```python
from build123d import *

# Parameters (mm, degrees)
BOSS_EXTRUDE1_DEPTH      = 115
CUT_EXTRUDE3_START       = -15
CUT_EXTRUDE3_DEPTH       = 15
CUT_EXTRUDE4_DEPTH       = 67
SKETCH5_W                = 33
SKETCH5_H                = 40
CUT_EXTRUDE5_DEPTH       = 67
SKETCH6_W                = 40
SKETCH6_H                = 15
BOSS_EXTRUDE2_DEPTH      = 5
SKETCH7_W                = 15
SKETCH7_H                = 15
BOSS_EXTRUDE4_DEPTH      = 10
SKETCH8_W                = 7
SKETCH8_H                = 15
BOSS_EXTRUDE5_DEPTH      = 5
BOSS_EXTRUDE6_DEPTH      = 5
BOSS_EXTRUDE6_DEPTH_BACK = 15
SKETCH9_W                = 40
SKETCH9_H                = 15


with BuildPart() as part:
    # Sketch1 → Boss-Extrude1 (new body)
    with BuildSketch(Plane(origin=(0, 0, 0), x_dir=(0, 0, -1), z_dir=(1, 0, 0))):
        with BuildLine():
            Line((-10, 54.083269132), (-10, -1.916730868))
            ThreePointArc((-10, -1.916730868), (-7.071067812, -8.98779868), (0, -11.916730868))
            Line((0, -11.916730868), (20, -11.916730868))
            Line((20, -11.916730868), (20, -26.916730868))
            Line((20, -26.916730868), (-20, -26.916730868))
            Line((-20, -26.916730868), (-20, -51.23475383))
            ThreePointArc((-20, -51.23475383), (-54.753734942, 5.198895061), (-10, 54.083269132))
        make_face()
    extrude(amount=BOSS_EXTRUDE1_DEPTH)

    # Sketch2 → Cut-Extrude3 (cut)
    with BuildSketch(Plane(origin=(115, 0, 0), x_dir=(0, 0, -1), z_dir=(1, 0, 0)).offset(CUT_EXTRUDE3_START)):
        with BuildLine():
            Line((20, -21.916730868), (-54.666698166, -6.045834235))
            ThreePointArc((-54.666698166, -6.045834235), (-45.878767393, 34.080884973), (-10, 54.083269132))
            Line((-10, 54.083269132), (-10, -1.916730868))
            ThreePointArc((-10, -1.916730868), (-7.071067812, -8.98779868), (0, -11.916730868))
            Line((0, -11.916730868), (20, -11.916730868))
            Line((20, -11.916730868), (20, -21.916730868))
        make_face()
    extrude(amount=CUT_EXTRUDE3_DEPTH, mode=Mode.SUBTRACT)

    # Sketch4 → Cut-Extrude4 (cut)
    with BuildSketch(Plane(origin=(0, -11.916730868, 0), x_dir=(1, 0, 0), z_dir=(0, 1, 0))):
        with BuildLine():
            Line((10, 15), (90, 15))
            ThreePointArc((90, 15), (95, 10), (90, 5))
            Line((90, 5), (10, 5))
            ThreePointArc((10, 5), (5, 10), (10, 15))
        make_face()
    extrude(amount=-CUT_EXTRUDE4_DEPTH, mode=Mode.SUBTRACT)

    # Sketch5 → Cut-Extrude5 (cut)
    with BuildSketch(Plane(origin=(0, 0, 10), x_dir=(-1, 0, 0), z_dir=(0, 0, -1))):
        with Locations((-53.5, 34.083269132)):
            Rectangle(SKETCH5_W, SKETCH5_H)
    extrude(amount=-CUT_EXTRUDE5_DEPTH, mode=Mode.SUBTRACT)

    # Sketch6 → Boss-Extrude2 (add)
    with BuildSketch(Plane(origin=(0, 0, 10), x_dir=(-1, 0, 0), z_dir=(0, 0, -1))):
        with Locations((-17, 31.583269132)):
            Rectangle(SKETCH6_W, SKETCH6_H)
    extrude(amount=BOSS_EXTRUDE2_DEPTH)

    # Sketch7 → Boss-Extrude4 (add)
    with BuildSketch(Plane.ZY):
        with Locations((17.5, 31.583269132)):
            Rectangle(SKETCH7_W, SKETCH7_H)
    extrude(amount=BOSS_EXTRUDE4_DEPTH)

    # Sketch8 → Boss-Extrude5 (add)
    with BuildSketch(Plane(origin=(0, 0, 10), x_dir=(-1, 0, 0), z_dir=(0, 0, -1))):
        with Locations((6.5, 31.583269132)):
            Rectangle(SKETCH8_W, SKETCH8_H)
    extrude(amount=BOSS_EXTRUDE5_DEPTH)

    # Sketch9 → Boss-Extrude6 (add, two sides: drawn at the far end of the back side and taken through both)
    with BuildSketch(Plane(origin=(0, 0, 10), x_dir=(-1, 0, 0), z_dir=(0, 0, -1)).offset(-BOSS_EXTRUDE6_DEPTH_BACK)):
        with Locations((-90, 31.583269132)):
            Rectangle(SKETCH9_W, SKETCH9_H)
    extrude(amount=BOSS_EXTRUDE6_DEPTH + BOSS_EXTRUDE6_DEPTH_BACK)


solid = part.part
```
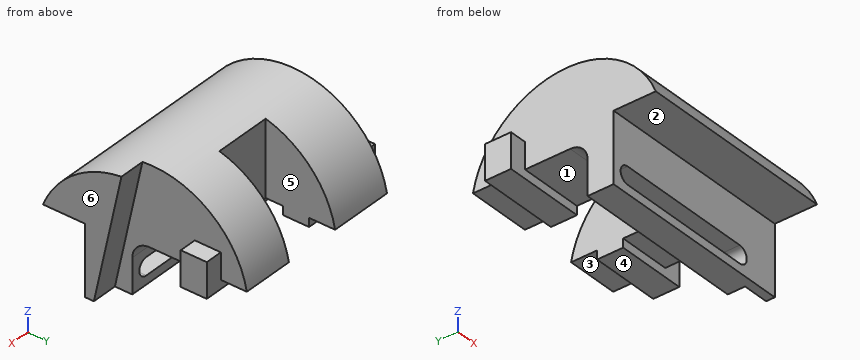
Verification items for the finished model (mm, model axes). Face numbers are marked on the shaded views. A direction names the side the tool comes from. Give positions to 0.01 mm unless a question says otherwise; leave off trailing zeros. Order: outer loops, then holes, each group sorted by start corner. A loop starts at its lowest first (then second) coordinate and runs counter-clockwise, first axis right, second up. Notation, with made-up numbers: M -30,-22 L -24,-22 A17 ccw -24,1 Z; hole C 85,7.25 d10. An arc over 180 degrees is marked long. Return JSON: item names as keys, results as strings. Group by question number.
1) Section check A-A on x = 105.5. Record the cut outline in (y, z).
2) Mould release check, pull along X, two halves, no side actions. Record for the marked faces 4, 5 and 6: pulls with the +X half, pulls with the -X half, needs draft (parallel to the pull), parting line crosses it, or undercut.
3) Go/stop test with flat-tipped pins: pin 1 Ø12 at (x, y) = (78.5, 46.5) entering from -Z; pin 2 Ø10 at (x, y) = (37.5, 28.5) entering from +Z; pin 3 Ø10 at (x, z) = (86, 14.5) entering from -Y. Record where each tip stops, or that it passes through.
4) Access from +Z, -Z, +X, -X, +Y, -Y to the whole of each face (thin tool, end or side, straight path). Record for the marked faces 1, 2 and 3.
5) Section check B-B on x = 84. Record the cut outline in (y, z), and give its area (3 significant figures).
6) Section check D-D on y = 26. Record the cut outline in (x, z), and give its area (3 significant figures).
7) Scan lines: line 1 (X direction, y = 25.5, z = 13.5); line 2 (X direction, y = 28.5, z = 34.5); line 3 (X direction, y = -16, z = 47). Record each from-to range of solid material in increasing order.
8) Section check C-C on z = -10. Record the cut outline in (x, y), and give its area (3 significant figures).
Answer block:
{
 "1": {"outline": "M -51.23,20 L -26.92,20 L -26.92,-20 L -21.92,-20 L -6.05,54.67 A55 ccw Z; M 24.08,5 L 39.08,5 L 39.08,25 L 24.08,25 Z"},
 "2": {"face 4": "needs draft", "face 5": "undercut", "face 6": "pulls with the +X half"},
 "3": {"pin 1": "stops at z = 10", "pin 2": "stops at z = 49.71", "pin 3": "stops at y = -26.92"},
 "4": {"face 1": "-Z, +X, -X", "face 2": "-Z, +X, -X, -Y", "face 3": "-Z, +X, -X, +Y"},
 "5": {"outline": "M -51.23,20 L -26.92,20 L -26.92,-5 L -11.92,-5 L -11.92,0 A10 cw -1.92,10 L 24.08,10 L 24.08,5 L 39.08,5 L 39.08,10 L 54.08,10 A55 ccw Z; M -26.92,-20 L -11.92,-20 L -11.92,-15 L -26.92,-15 Z", "area": "3,800 mm^2"},
 "6": {"outline": "M -10,5 L 37,5 L 37,48.47 L 0,48.47 L 0,25 L -10,25 Z; M 70,5 L 110,5 L 110,25 L 100,25 L 100,48.47 L 70,48.47 Z", "area": "3,310 mm^2"},
 "7": {"line 1": "x = -10 to 37, 70 to 110", "line 2": "x = 0 to 37, 70 to 100", "line 3": "x = 0 to 115"},
 "8": {"outline": "M 0,-26.92 L 5,-26.92 L 5,-11.92 L 0,-11.92 Z; M 95,-26.92 L 115,-26.92 L 115,-19.79 L 100,-19.79 L 100,-11.92 L 95,-11.92 Z", "area": "257 mm^2"}
}
